```python
from build123d import *

# Parameters (mm, degrees)
SKETCH1_R           = 1.75
SKETCH1_W           = 110
SKETCH1_H           = 150
BOSS_EXTRUDE1_DEPTH = 0.5


with BuildPart() as part:
    # Sketch1 → Boss-Extrude1 (new body)
    with BuildSketch(Plane.XY):
        with BuildLine():
            Line((60, -85), (-60, -85))
            ThreePointArc((-60, -85), (-63.535533906, -83.535533906), (-65, -80))
            Line((-65, -80), (-65, 80))
            ThreePointArc((-65, 80), (-63.535533906, 83.535533906), (-60, 85))
            Line((-60, 85), (60, 85))
            ThreePointArc((60, 85), (63.535533906, 83.535533906), (65, 80))
            Line((65, 80), (65, -80))
            ThreePointArc((65, -80), (63.535533906, -83.535533906), (60, -85))
        make_face()
        with Locations((60, -27)):
            Circle(SKETCH1_R, mode=Mode.SUBTRACT)
        with Locations((60, -80)):
            Circle(SKETCH1_R, mode=Mode.SUBTRACT)
        with Locations(Location((-60, -27, 0), (0, 0, 180))):
            Circle(SKETCH1_R, mode=Mode.SUBTRACT)
        with Locations(Location((-60, -80, 0), (0, 0, 180))):
            Circle(SKETCH1_R, mode=Mode.SUBTRACT)
        with Locations((0, -80)):
            Circle(SKETCH1_R, mode=Mode.SUBTRACT)
        with Locations(Location((60, 27, 0), (0, 0, 180))):
            Circle(SKETCH1_R, mode=Mode.SUBTRACT)
        with Locations(Location((60, 80, 0), (0, 0, 180))):
            Circle(SKETCH1_R, mode=Mode.SUBTRACT)
        with Locations(Location((0, 80, 0), (0, 0, 180))):
            Circle(SKETCH1_R, mode=Mode.SUBTRACT)
        with Locations((-60, 27)):
            Circle(SKETCH1_R, mode=Mode.SUBTRACT)
        with Locations((-60, 80)):
            Circle(SKETCH1_R, mode=Mode.SUBTRACT)
        Rectangle(SKETCH1_W, SKETCH1_H, mode=Mode.SUBTRACT)
    extrude(amount=BOSS_EXTRUDE1_DEPTH)


solid = part.part
```
Check sheet for the modelled part. Datum: model origin and axes. Units: mm. Round coordinates to 2 decimals unless told otherwise and drop trailing zeros. Loops run counter-clockwise (first coordinate to the right, second up) from the corner with the lowest first, then second, coordinate; pieces in that order, holes last. Notation, with made-up numbers: (79, 70.5) - (97, 70.5) arc R18 ccw to (97, 105.5) - close; hole circle Ø5 at (-0.5, 3). An arc over 180 degrees is marked (long way). Answer as a JSON object with one key per item and string values. Group by question number.
Q1. Sectioned sample at C-C, the plane x = -17. Enter the section's corners in (y, z).
Q2. Mould release check, pull along X, two halves, no side actions. Record for faces 1 (the face through (-63.57, 83.5, 0.25)), 2 (the face through (58, 0, 0)), 3 (the face through (-61.617, -79.33, 0.246)), 4 (the face through (63.57, -83.5, 0.25)): released by +X, released by -X, zero draft, split by the parting line, or undercut.
Q3. Scan lines: line 1 along Y through (x, z) = (60, 0.25); line 2 along X through (y, z) = (80, 0.35); line 3 along Y through (x, z) = (-13, 0.05). Record each from-to range of solid material in increasing order. Write a range as [from, to].
Q4. Sectioned sample at D-D, the plane y = -27. Enter the section's corners in (x, z), plus the area to 3 significant figures.
Q5. Sectioned sample at B-B, the plane y = 55. Enter the section's corners in (x, z), plus the area to 3 significant figures.
Q6. Sectioned sample at A-A, the plane x = 0. Enter the section's corners in (y, z), plus the area to 3 significant figures.
Solution:
{
 "1": {"outline": "(-85, 0) - (-75, 0) - (-75, 0.5) - (-85, 0.5) - close; (75, 0) - (85, 0) - (85, 0.5) - (75, 0.5) - close"},
 "2": {"face 1": "released by -X", "face 2": "zero draft", "face 3": "undercut", "face 4": "released by +X"},
 "3": {"line 1": "y = [-85, -81.75], [-78.25, -28.75], [-25.25, 25.25], [28.75, 78.25], [81.75, 85]", "line 2": "x = [-65, -61.75], [-58.25, -1.75], [1.75, 58.25], [61.75, 65]", "line 3": "y = [-85, -75], [75, 85]"},
 "4": {"outline": "(-65, 0) - (-61.75, 0) - (-61.75, 0.5) - (-65, 0.5) - close; (-58.25, 0) - (-55, 0) - (-55, 0.5) - (-58.25, 0.5) - close; (55, 0) - (58.25, 0) - (58.25, 0.5) - (55, 0.5) - close; (61.75, 0) - (65, 0) - (65, 0.5) - (61.75, 0.5) - close", "area": "6.50 mm²"},
 "5": {"outline": "(-65, 0) - (-55, 0) - (-55, 0.5) - (-65, 0.5) - close; (55, 0) - (65, 0) - (65, 0.5) - (55, 0.5) - close", "area": "10.0 mm²"},
 "6": {"outline": "(-85, 0) - (-81.75, 0) - (-81.75, 0.5) - (-85, 0.5) - close; (-78.25, 0) - (-75, 0) - (-75, 0.5) - (-78.25, 0.5) - close; (75, 0) - (78.25, 0) - (78.25, 0.5) - (75, 0.5) - close; (81.75, 0) - (85, 0) - (85, 0.5) - (81.75, 0.5) - close", "area": "6.50 mm²"}
}
